Here's the drawing with two shaded views (mm, measured from the low corner). I have some questions. Coordinates: 2 decimals unless noted, no trailing zeros. Loops run counter-clockwise (first coordinate to the right, second up) from the corner with the lowest first, then second, coordinate; pieces in that order, holes last. Notation, with made-up numbers: (74, -4.75) - (110, -4.75) arc R25 cw to (110, 34.25) - close; hole circle Ø8 at (-24, 38). An arc over 180 degrees is marked (long way). One line per item, written item: value. Start each with the question number.
(1) If we section it at B-B on z = 8: Write out the boundary of the cut face in (x, y).
(2) If we section it at A-A on x = 3: Write out the boundary of the cut face in (y, z).
(3) If I drill on line 1 along X through (y, z) = (1.9, 8); line 2 along Z through (x, y) = (3, 2.1); line 3 along X through (y, z) = (3.5, 9.25), over which ranges is the centre line in solid material (lowest first)? Write a range as from..to.
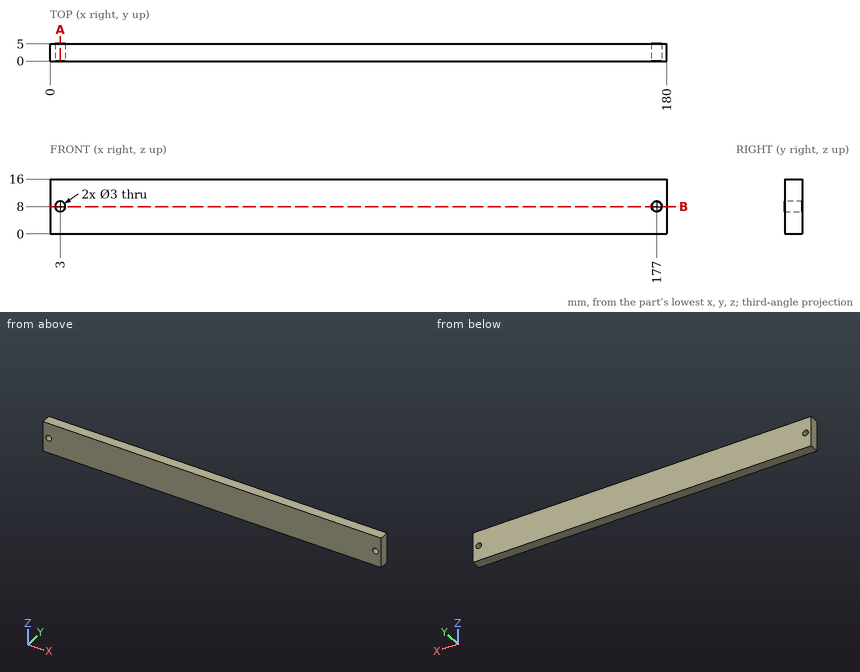
Values:
1. outline: (0, 0) - (1.5, 0) - (1.5, 5) - (0, 5) - close; (4.5, 0) - (175.5, 0) - (175.5, 5) - (4.5, 5) - close; (178.5, 0) - (180, 0) - (180, 5) - (178.5, 5) - close
2. outline: (0, 0) - (5, 0) - (5, 6.5) - (0, 6.5) - close; (0, 9.5) - (5, 9.5) - (5, 16) - (0, 16) - close
3. line 1: x = 0..1.5, 4.5..175.5, 178.5..180
3. line 2: z = 0..6.5, 9.5..16
3. line 3: x = 0..2.17, 3.83..176.17, 177.83..180
